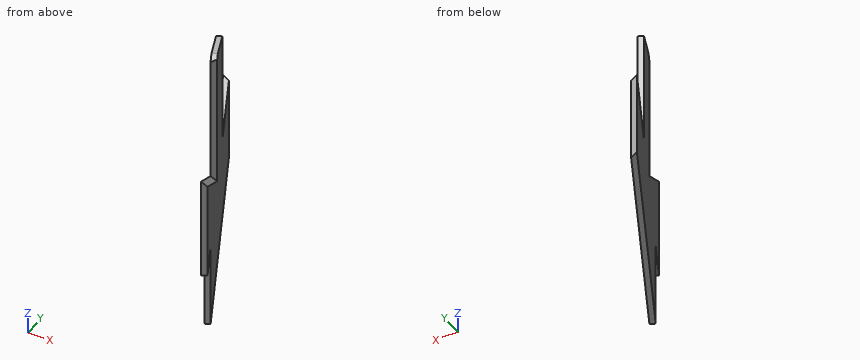
from build123d import *

# Parameters (mm, degrees)
BOSS_EXTRUDE1_DEPTH = 208.295834
CUT_EXTRUDE1_DEPTH  = 233.9651465
CUT_EXTRUDE3_DEPTH  = 106.39675924
BOSS_EXTRUDE2_DEPTH = 79


with BuildPart() as part:
    # Sketch2 → Boss-Extrude1 (new body)
    with BuildSketch(Plane.XY.offset(133.323635178)):
        Polygon((-552.096326618, 302.497295421), (-547.608266937, 304.701228339), (-659.457001573, 532.468503885), (-662.259879772, 526.832889814), align=None)
    extrude(amount=BOSS_EXTRUDE1_DEPTH)

    # Sketch3 → Cut-Extrude1 (cut, through all)
    with BuildSketch(Plane(origin=(56.456528708, 113.514460847, 99.05047984), x_dir=(-0.935748975, 0.239556806, 0.258817295), z_dir=(-0.350913088, -0.705564279, -0.615661475))):
        Polygon((641.877398582, 324.891396181), (520.568005211, 262.71812893), (690.075774021, -224.74438404), (811.385167392, -162.571116789), align=None)
    extrude(amount=-CUT_EXTRUDE1_DEPTH, mode=Mode.SUBTRACT)

    # Sketch5 → Cut-Extrude3 (cut, through all)
    with BuildSketch(Plane(origin=(-325.143320908, -159.666786774, 0), x_dir=(0, 0, 1), z_dir=(-0.897611936, -0.440786584, 0))):
        Polygon((263.823635178, 620.544936833), (263.823635178, 631.781992675), (239.430319814, 682.249402309), (133.323635178, 682.249402309), (133.323635178, 768.6298834), (341.619468978, 768.6298834), (341.619468978, 620.544936833), align=None)
    extrude(amount=-CUT_EXTRUDE3_DEPTH, mode=Mode.SUBTRACT)

    # Sketch6 → Boss-Extrude2 (add)
    with BuildSketch(Plane(origin=(0, 0, 133.323635178), x_dir=(-1, 0, 0), z_dir=(0, 0, -1))):
        Polygon((567.701533334, 334.275530817), (563.213473653, 336.479463735), (653.626470855, 520.595288681), (660.996902767, 524.260980239), align=None)
    extrude(amount=BOSS_EXTRUDE2_DEPTH)


solid = part.part
Read the model definition and answer for the solid it produces. Units are mm, in the model's axes. Round coordinates to 2 decimals unless told otherwise and drop trailing zeros. Write each loop counter-clockwise with the first axis right and the second up, starting at its lowest first coordinate (ties: lowest second). Pieces come first, ordered by that corner, then holes. Notation, with made-up numbers: (-26, 5.25) - (19, 5.25) arc R27 ccw to (19, 32.25) - close; hole circle Ø11 at (41, 25.25). An arc over 180 degrees is marked (long way). Use a Markdown table: item, result.
(1) The part is cut by section A-A (z = 174.5). Write down the section's boundary in (x, y).
Reported:
| item | result |
|---|---|
| outline | (-625.87, 452.73) - (-598.67, 397.34) - (-595.87, 402.98) - (-621.38, 454.93) - close; (-583.18, 365.8) - (-552.1, 302.5) - (-547.61, 304.7) - (-575.81, 362.14) - close |
(2) Straight lines are drawn through the part: line 1 along Y through (x, z) = (-641.5, 117.5); line 2 along X through (y, z) = (350, 156); line 3 along Y through (x, z) = (-644, 71). For each, find the intervals that lie inside material, in ascending order. Write a range as [from, to].
Reported:
| item | result |
|---|---|
| line 1 | [484.56, 495.9] |
| line 2 | [-575.42, -569.85] |
| line 3 | [489.65, 500.99] |
(3) The part is cut by section B-B (z = 197.5). Write down the section's boundary in (x, y), then the cut area to 3 significant figures.
Reported:
| item | result |
|---|---|
| outline | (-625.87, 452.73) - (-598.67, 397.34) - (-595.87, 402.98) - (-621.38, 454.93) - close; (-570.14, 339.25) - (-552.1, 302.5) - (-547.61, 304.7) - (-562.77, 335.58) - close |
| area | 487 mm2 |
(4) The part is cut by section D-D (x = -641). Write down the section's boundary in (y, z).
Reported:
| item | result |
|---|---|
| outline | (483.54, 54.32) - (494.88, 54.32) - (494.88, 133.32) - (483.54, 133.32) - close |
(5) The part is cut by section C-C (y = 327). Write down the section's boundary in (x, z), then the cut area to 3 significant figures.
Reported:
| item | result |
|---|---|
| outline | (-564.13, 133.32) - (-558.56, 133.32) - (-558.56, 204.94) - (-564.13, 208.11) - close |
| area | 408 mm2 |
(6) Each of these flat-tipped pins is pushed along its axis until it touches: pin 1 Ø8 at (y, z) = (469.5, 79.5) entering from -X; pin 2 Ø1.5 at (x, z) = (-599, 138.5) entering from -Y; pin 3 Ø3 at (x, z) = (-604.5, 119.5) entering from +Y. Where does it stop, or does it pass through?
Reported:
| item | result |
|---|---|
| pin 1 | x = -636.07 |
| pin 2 | y = 396.48 |
| pin 3 | y = 423.61 |
